```python
from build123d import *

# Parameters (mm, degrees)
MODEL_R                  = 1.8
MODEL_R_2                = 4.1
MODEL_W                  = 7.7
MODEL_H                  = 6.9
RESSALTO_EXTRUS_O1_DEPTH = 6


with BuildPart() as part:
    # Model → Ressalto-extrusão1 (new body)
    with BuildSketch(Plane.XY):
        Polygon((52.383398063, 73.075042987), (52.28349764, 72.833862032), (52.249423467, 72.575042987), (52.249423467, 67.575042987), (42.750846371, 67.575042987), (42.750846371, 72.575042987), (42.716772197, 72.833862032), (42.616871774, 73.075042987), (42.457953152, 73.282149768), (42.250846371, 73.441068391), (42.009665416, 73.540968814), (41.750846371, 73.575042987), (39.151153585, 73.575042987), (38.89233454, 73.540968814), (38.651153585, 73.441068391), (38.444046804, 73.282149768), (38.285128182, 73.075042987), (38.185227759, 72.833862032), (38.151153585, 72.575042987), (38.151153585, 67.575042987), (30.849423467, 67.575042987), (30.849423467, 48.514129082), (27.849423467, 45.514129082), (27.849423467, 41.05308967), (27.845731051, 41.025042987), (27.849423467, 40.996996305), (27.849423467, 36.535956893), (30.849423467, 33.535956893), (30.849423467, 14.475042987), (38.151153585, 14.475042987), (38.155087445, 9.474256339), (38.189331183, 9.215590795), (38.289324067, 8.974588885), (38.448258531, 8.767658139), (38.655314239, 8.608886505), (38.896394733, 8.509083236), (39.155087136, 8.475042987), (41.749423467, 8.475042987), (42.008242512, 8.509117161), (42.249423467, 8.609017584), (42.456530248, 8.767936206), (42.61544887, 8.975042987), (42.715349293, 9.216223942), (42.749423467, 9.475042987), (42.749423467, 14.475042987), (52.249423467, 14.475042987), (52.249423467, 9.475042987), (52.28349764, 9.216223942), (52.383398063, 8.975042987), (52.542316685, 8.767936206), (52.749423467, 8.609017584), (52.990604422, 8.509117161), (53.249423467, 8.475042987), (74.549423467, 8.475042987), (74.808242512, 8.509117161), (75.049423467, 8.609017584), (75.256530248, 8.767936206), (75.41544887, 8.975042987), (75.515349293, 9.216223942), (75.549423467, 9.475042987), (75.549423467, 14.475042987), (86.849423467, 14.475042987), (86.849423467, 67.575042987), (75.549423467, 67.575042987), (75.549423467, 72.575042987), (75.515349293, 72.833862032), (75.41544887, 73.075042987), (75.256530248, 73.282149768), (75.049423467, 73.441068391), (74.808242512, 73.540968814), (74.549423467, 73.575042987), (53.249423467, 73.575042987), (52.990604421, 73.540968814), (52.749423467, 73.441068391), (52.542316685, 73.282149768), align=None)
        with Locations((81.849423467, 18.525042987)):
            Circle(MODEL_R, mode=Mode.SUBTRACT)
        with Locations((39.849423467, 24.575042987)):
            Circle(MODEL_R, mode=Mode.SUBTRACT)
        with Locations((35.849423467, 41.025042987)):
            Circle(MODEL_R_2, mode=Mode.SUBTRACT)
        with Locations((39.849423467, 57.475042987)):
            Circle(MODEL_R, mode=Mode.SUBTRACT)
        with Locations((81.849423467, 63.525042987)):
            Circle(MODEL_R, mode=Mode.SUBTRACT)
        Polygon((58.966889554, 29.175042987), (58.966889554, 52.875042987), (51.598425396, 52.875042987), (51.598425396, 59.775042987), (58.966889554, 59.775042987), (58.966889554, 66.025032836), (69.966884557, 66.025032836), (69.966884557, 16.025053138), (58.966889554, 16.025053138), (58.966889554, 22.275042987), (51.598425396, 22.275042987), (51.598425396, 29.175042987), align=None, mode=Mode.SUBTRACT)
        with Locations((78.516884557, 56.325042987)):
            Rectangle(MODEL_W, MODEL_H, mode=Mode.SUBTRACT)
        with Locations((78.516884557, 25.725042987)):
            Rectangle(MODEL_W, MODEL_H, mode=Mode.SUBTRACT)
    extrude(amount=RESSALTO_EXTRUS_O1_DEPTH)


solid = part.part
```
Verification items for the finished model (mm, model axes). A direction names the side the tool comes from. Coordinates: 2 decimals unless noted, no trailing zeros. Loops run counter-clockwise (first coordinate to the right, second up) from the corner with the lowest first, then second, coordinate; pieces in that order, holes last. Notation, with made-up numbers: (18.25, -22.5) -> (29.25, -22.5) arc R24 cw to (29.25, 2.5) -> close; hole circle Ø3 at (-19, 73.5). An arc over 180 degrees is marked (long way). Answer in a Markdown table with one row per item.
1) Access from +Z, -Z, +X, -X, +Y, -Y to the whole of each face (thin tool, end or side, straight path). Record for faces 5 (the face through (75.549, 70, 3)), 6 (the face through (42.749, 12, 3)), 7 (the face through (58.967, 41, 3)).
The answers:
| item | result |
|---|---|
| face 5 | +Z, -Z, +X, +Y |
| face 6 | +Z, -Z, -Y |
| face 7 | +Z, -Z |
2) Depth check by flat-ended pin: P1, Ø1.3, axis at y = 42.5, z = 4, coming from the -X side; P2, Ø3, axis at x = 35, z = 4, coming from the +Y side; P3, Ø1.5, axis at y = 11, z = 3.5, coming from the -X side; P4, Ø12, axis at x = 39.5, y = 29.5, coming from the -Z side. Enter the tip coordinate at first touch or a pass-through.
The answers:
| item | result |
|---|---|
| P1 | stops at x = 27.85 |
| P2 | stops at y = 67.58 |
| P3 | stops at x = 38.15 |
| P4 | stops at z = 0 |
3) Section check B-B (y = 32). Record the cut outline in (x, z).
The answers:
| item | result |
|---|---|
| outline | (30.85, 0) -> (58.97, 0) -> (58.97, 6) -> (30.85, 6) -> close; (69.97, 0) -> (86.85, 0) -> (86.85, 6) -> (69.97, 6) -> close |
4) Section check A-A (x = 77). Record the cut outline in (y, z), and give its area (3 significant figures).
The answers:
| item | result |
|---|---|
| outline | (14.48, 0) -> (22.28, 0) -> (22.28, 6) -> (14.48, 6) -> close; (29.18, 0) -> (52.88, 0) -> (52.88, 6) -> (29.18, 6) -> close; (59.78, 0) -> (67.58, 0) -> (67.58, 6) -> (59.78, 6) -> close |
| area | 236 mm2 |
5) Draft check along Y on faces 1 (the face through (74.667, 56, 3)), 2 (the face through (81, 14.475, 3)), 3 (the face through (29.37, 47.035, 2.958)), 4 (the face through (65, 16.025, 3)). Enter one of: released by +Y, released by -Y, zero draft, split by the parting line, or undercut.
The answers:
| item | result |
|---|---|
| face 1 | undercut |
| face 2 | released by -Y |
| face 3 | released by +Y |
| face 4 | undercut |
6) Section check C-C (x = 33.5). Record the cut outline in (y, z).
The answers:
| item | result |
|---|---|
| outline | (14.48, 0) -> (37.66, 0) -> (37.66, 6) -> (14.48, 6) -> close; (44.39, 0) -> (67.58, 0) -> (67.58, 6) -> (44.39, 6) -> close |
7) Section check D-D (x = 56). Record the cut outline in (y, z).
The answers:
| item | result |
|---|---|
| outline | (8.48, 0) -> (22.28, 0) -> (22.28, 6) -> (8.48, 6) -> close; (29.18, 0) -> (52.88, 0) -> (52.88, 6) -> (29.18, 6) -> close; (59.78, 0) -> (73.58, 0) -> (73.58, 6) -> (59.78, 6) -> close |
8) Scan lines: line 1 along Y through (x, z) = (54, 2.15); line 2 along X through (y, z) = (28, 1.6); line 3 along X through (y, z) = (65.5, 0.75). Record each from-to range of solid material in increasing order. Write a range as from..to.
The answers:
| item | result |
|---|---|
| line 1 | y = 8.48..22.28, 29.18..52.88, 59.78..73.58 |
| line 2 | x = 30.85..51.6, 69.97..74.67, 82.37..86.85 |
| line 3 | x = 30.85..58.97, 69.97..86.85 |
